from build123d import *

# Parameters (mm, degrees)
SKETCH_R     = 14
PAD_DEPTH    = 25
SKETCH001_W  = 34
SKETCH001_H  = 32
PAD001_DEPTH = 11
SKETCH002_R  = 10
PAD002_DEPTH = 9
SKETCH003_R  = 8
PAD003_DEPTH = 3
PAD004_DEPTH = 12
SKETCH005_R  = 1.75
POCKET_DEPTH = 100


with BuildPart() as part:
    # Sketch → Pad (new body)
    with BuildSketch(Plane.YZ):
        Circle(SKETCH_R)
    extrude(amount=-PAD_DEPTH)

    # Sketch001 (on Face2 of Pad) → Pad001 (join)
    with BuildSketch(Plane.YZ):
        Rectangle(SKETCH001_W, SKETCH001_H)
    extrude(amount=PAD001_DEPTH)

    # Sketch002 (on Face5 of Pad001) → Pad002 (join)
    with BuildSketch(Plane.YZ.offset(11)):
        Circle(SKETCH002_R)
    extrude(amount=PAD002_DEPTH)

    # Sketch003 (on Face10 of Pad002) → Pad003 (join)
    with BuildSketch(Plane.YZ.offset(20)):
        Circle(SKETCH003_R)
    extrude(amount=PAD003_DEPTH)

    # Sketch004 (on Face12 of Pad003) → Pad004 (join)
    with BuildSketch(Plane.YZ.offset(23)):
        Polygon((0, 4.041452), (-3.5, 2.020726), (-3.5, -2.020726), (0, -4.041452), (3.5, -2.020726), (3.5, 2.020726), align=None)
    extrude(amount=PAD004_DEPTH)

    # Sketch005 (on Face1 of Pad004) → Pocket (cut)
    with BuildSketch(Plane(origin=(0, 0, 16), x_dir=(0, -1, 0), z_dir=(0, 0, 1))):
        with Locations((-14.15, 3)):
            Circle(SKETCH005_R)
        with Locations((14.15, 3)):
            Circle(SKETCH005_R)
    extrude(amount=-POCKET_DEPTH, mode=Mode.SUBTRACT)


solid = part.part
The model under review builds one solid part; all positions refer to its coordinate system, in mm. A direction names the side the tool comes from. Give positions to 0.01 mm unless a question says otherwise; leave off trailing zeros. Loops run counter-clockwise (first coordinate to the right, second up) from the corner with the lowest first, then second, coordinate; pieces in that order, holes last. Notation, with made-up numbers: (-15.5, 70.25) -> (38.5, 70.25) arc R16 ccw to (38.5, 76.25) -> close; hole circle Ø11 at (-27, 48.25). An arc over 180 degrees is marked (long way). Put each result on its own line as item: value. Start each with the question number.
1. We need section B-B on x = 3. State the section outline as (y, z) points.
2. We need section C-C on y = -1. State the section outline as (x, z) points, then the cut area to 3 significant figures.
3. Mouldability with a two-part tool opening along Y and no side actions: class faces 1 (the face through (29, 3.5, 0)), 2 (the face through (5, 0, 16)), 3 (the face through (2.33, 12.533, 0.224)), 4 (the face through (28.916, -1.726, 3.045)) as released by +Y, released by -Y, zero draft, split by the parting line, or undercut.
4. Clearance check with flat-ended pins moving along their axes: P1, Ø6, axis at y = 7.5, z = -6, coming from the +X side; P2, Ø6, axis at y = -8.5, z = 9.5, coming from the +X side; P3, Ø12, axis at x = -13, z = -11.5, coming from the +Y side; P4, Ø4.5, axis at x = 3, y = 14.15, coming from the +Z side. State where each tip first meets the part, or that it passes through.
5. For faces 5 (the face through (28.9, 1.8, 3)), 6 (the face through (20, 0, 8.2)), 7 (the face through (28.9, -1.8, -3)), 8 (the face through (-12.325, 12.932, -5.362)), 9 (the face through (28.916, 1.726, -3.045)), list the 3-axis set-ups (+Z, -Z, +X, -X, +Y, -Y) from which the entire face can be reached by the end or side of a thin tool; tool diameter is ignored.
6. Wall thickness on probe 1 along X at (y, z) = (-14.15, 1.5); probe 2 along Y at (x, z) = (3.5, 6.5); probe 3 along Z at (x, y) = (-4, 0): over which ranges is each line inside the solid? List them lowest first.
7. We need section D-D on x = 14. State the section outline as (y, z) points, then the cut area to 3 significant figures.
8. We need section A-A on z = 0. State the section outline as (x, y) points.
Determined:
1. outline: (-17, -16) -> (-15.9, -16) -> (-15.9, 16) -> (-17, 16) -> close; (-12.4, -16) -> (12.4, -16) -> (12.4, 16) -> (-12.4, 16) -> close; (15.9, -16) -> (17, -16) -> (17, 16) -> (15.9, 16) -> close
2. outline: (-25, -13.96) -> (0, -13.96) -> (0, -16) -> (11, -16) -> (11, -9.95) -> (20, -9.95) -> (20, -7.94) -> (23, -7.94) -> (23, -3.46) -> (35, -3.46) -> (35, 3.46) -> (23, 3.46) -> (23, 7.94) -> (20, 7.94) -> (20, 9.95) -> (11, 9.95) -> (11, 16) -> (0, 16) -> (0, 13.96) -> (-25, 13.96) -> close
2. area: 1,360 mm^2
3. face 1: released by +Y
3. face 2: zero draft
3. face 3: undercut
3. face 4: released by -Y
4. P1: x = 23
4. P2: x = 20
4. P3: y = 12.87
4. P4: z = 16
5. face 5: +Z, +X, +Y
5. face 6: +X
5. face 7: -Z, +X, -Y
5. face 8: -X
5. face 9: -Z, +X, +Y
6. probe 1: 0 to 1.25, 4.75 to 11
6. probe 2: -17 to -15.83, -12.47 to 12.47, 15.83 to 17
6. probe 3: -14 to 14
7. outline: circle Ø20 at (0, 0)
7. area: 314 mm^2
8. outline: (-25, -14) -> (0, -14) -> (0, -17) -> (11, -17) -> (11, -10) -> (20, -10) -> (20, -8) -> (23, -8) -> (23, -3.5) -> (35, -3.5) -> (35, 3.5) -> (23, 3.5) -> (23, 8) -> (20, 8) -> (20, 10) -> (11, 10) -> (11, 17) -> (0, 17) -> (0, 14) -> (-25, 14) -> close; hole circle Ø3.5 at (3, -14.15); hole circle Ø3.5 at (3, 14.15)
